Autodesk Inventor part; units mm, degrees
ref_plane "YZ Plane" through (0, 0, 0) normal (1, 0, 0) x (0, 1, 0)
ref_plane "XZ Plane" through (0, 0, 0) normal (0, 1, 0) x (-1, 0, 0)
ref_plane "XY Plane" through (0, 0, 0) normal (0, 0, 1) x (1, 0, 0)
sketch "Sketch1" plane through (0, 0, 0) normal (0, 1, 0) x (-1, 0, 0)
  line L0 (0, 0) -> (-55.6345, 0)
  line L1 (-55.6345, 0) -> (-55.6345, 15.875)
  line L2 (-55.6345, 15.875) -> (0, 15.875)
  line L3 (0, 15.875) -> (0, 0)
  dimension "d0" = 55.6345
  dimension "d1" = 15.875
extrude "Extrusion1" add sketch "Sketch1" along normal blind 5.6134
sketch "Sketch7" plane through (0, 5.6134, 0) normal (0, 1, 0) x (1, 0, 0)
  circle A0 centre (9.3218, -6.6524) radius 1.6
  circle A1 centre (46.3218, -6.6524) radius 1.6
  line L0 (0, 0) -> (0, -15.875)
  line L1 (55.6345, 0) -> (0, 0)
  line L2 (55.6345, -15.875) -> (55.6345, 0)
  dimension "d22" = 3.2
  dimension "d23" = 3.2
  dimension "d24" = 37
  dimension "d43" = 6.6524
  dimension "d44" = 6.6524
  dimension "d48" = 9.3218
  dimension "d49" = 9.3127
extrude "Extrusion6" cut sketch "Sketch7" against normal blind 25.4
sketch "Sketch8" plane through (0, 5.6134, 0) normal (0, 1, 0) x (1, 0, 0)
  line L0 (55.6345, 0) -> (0, 0)
  line L1 (0, 0) -> (0, -15.875)
  line L2 (55.6345, -15.875) -> (55.6345, 0)
  line L3 (0, -15.875) -> (3.175, -15.875)
  line L4 (3.175, -15.875) -> (3.175, 0)
  line L5 (3.175, 0) -> (0, 0)
  line L6 (0, 0) -> (0, -15.875)
  line L7 (55.6345, -15.875) -> (52.4595, -15.875)
  line L8 (52.4595, -15.875) -> (52.4595, 0)
  line L9 (52.4595, 0) -> (55.6345, 0)
  line L10 (55.6345, 0) -> (55.6345, -15.875)
  dimension "d34" = 3.175
  dimension "d35" = 3.175
extrude "Extrusion7" cut sketch "Sketch8" against normal blind 2.4384
equation "\"d23\" = d22"
properties part number "Lidar Sensor Case Piece 3"
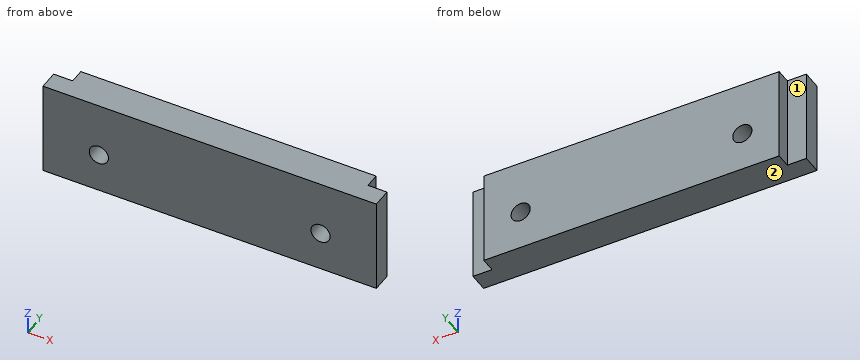
Source: CAD feature listing. Evaluate the final solid. Frame: model axes, mm. Face numbers are marked on the shaded views. A direction names the side the tool comes from. Coordinates: 2 decimals unless noted, no trailing zeros. Write each loop counter-clockwise with the first axis right and the second up, starting at its lowest first coordinate (ties: lowest second). Pieces come first, ordered by that corner, then holes. Notation, with made-up numbers: M -25.5,30.5 L 12.5,30.5 A24 cw 12.5,64.5 Z; hole C -21.5,20 d6. An arc over 180 degrees is marked long. Answer as a JSON object with one key per item and string values.
1. Cut plane B-B on z = 12.25. Output: boundary loops of the cut face in (x, y) (1 decimal).
Evaluation:
{"outline": "M 0,0 L 55.6,0 L 55.6,3.2 L 52.5,3.2 L 52.5,5.6 L 3.2,5.6 L 3.2,3.2 L 0,3.2 Z"}
2. Contact query for flat-ended pins moving along their axis: P1, Ø2, axis at y = 4.5, z = 11, coming from the +X side; P2, Ø1, axis at x = 54.5, z = 7.5, coming from the +Y side (3 decimals). Output: stop coordinate, or through.
Evaluation:
{"P1": "x = 52.46", "P2": "y = 3.175"}
3. Access query for the marked faces 1 and 2. Directions: +Z, -Z, +X, -X, +Y, -Y. A direction counts if a zero-diameter tool reaches every point of the face in a straight line with its end or side. Return the directions, or none.
Evaluation:
{"face 1": "+Z, -Z, -X, +Y", "face 2": "-Z, +X, -X, +Y, -Y"}
4. Cut plane C-C on y = 4.1. Output: boundary loops of the cut face in (x, z) (1 decimal).
Evaluation:
{"outline": "M 3.2,0 L 52.5,0 L 52.5,15.9 L 3.2,15.9 Z; hole C 9.3,6.7 d3.2; hole C 46.3,6.7 d3.2"}
5. Cut plane A-A on z = 7.25. Output: boundary loops of the cut face in (x, y) (1 decimal).
Evaluation:
{"outline": "M 0,0 L 7.8,0 L 7.8,5.6 L 3.2,5.6 L 3.2,3.2 L 0,3.2 Z; M 10.8,0 L 44.8,0 L 44.8,5.6 L 10.8,5.6 Z; M 47.8,0 L 55.6,0 L 55.6,3.2 L 52.5,3.2 L 52.5,5.6 L 47.8,5.6 Z"}
6. Ray query, L1, parallel to X at y = 5.25, z = 6.5 (1 decimal); L2, parallel to X at y = 0.95, z = 6.75; L3, parallel to X at y = 4.95, z = 13 (1 decimal). Return the intervals inside material, ascending.
Evaluation:
{"L1": "3.2 to 7.7, 10.9 to 44.7, 47.9 to 52.5", "L2": "0 to 7.72, 10.92 to 44.72, 47.92 to 55.63", "L3": "3.2 to 52.5"}
